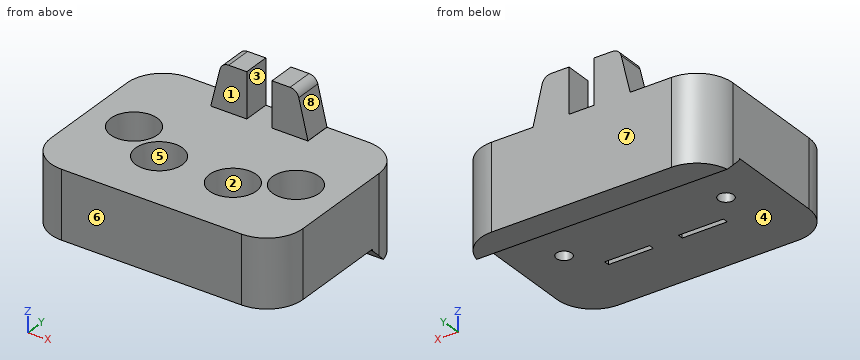
from build123d import *

# Parameters (mm, degrees)
SKETCH_W        = 35.56
SKETCH_H        = 25.4
SKETCH_R        = 1.0795
SKETCH_W_2      = 6.35
SKETCH_H_2      = 0.762
PAD_DEPTH       = 1.905
SKETCH001_W     = 35.56
SKETCH001_H     = 25.4
PAD001_DEPTH    = 7.62
SKETCH002_R     = 3.302
POCKET_DEPTH    = 7.62
SKETCH003_W     = 35.56
SKETCH003_H     = 6.35
PAD002_DEPTH    = 2.54
SKETCH004_W     = 5.08
SKETCH004_H     = 3.81
PAD003_DEPTH    = 6.35
CHAMFER_1_SIZE2 = 1.524
CHAMFER_1_SIZE  = 6.3246
CHAMFER_2_SIZE2 = 1.524
CHAMFER_2_SIZE  = 6.3246
FILLET_R        = 1.27
FILLET001_R     = 5.08
CHAMFER001_SIZE = 2.286


with BuildPart() as part:
    # Sketch → Pad (new body)
    with BuildSketch(Plane.XY):
        Rectangle(SKETCH_W, SKETCH_H)
        with Locations((-11.43, 0)):
            Circle(SKETCH_R, mode=Mode.SUBTRACT)
        with Locations((11.43, 0)):
            Circle(SKETCH_R, mode=Mode.SUBTRACT)
        with Locations((5.207, -4.191)):
            Rectangle(SKETCH_W_2, SKETCH_H_2, mode=Mode.SUBTRACT)
        with Locations((-5.207, -4.191)):
            Rectangle(SKETCH_W_2, SKETCH_H_2, mode=Mode.SUBTRACT)
    extrude(amount=PAD_DEPTH)

    # Sketch001 (on Face16 of Pad) → Pad001 (join)
    with BuildSketch(Plane.XY.offset(1.905)):
        Rectangle(SKETCH001_W, SKETCH001_H)
    extrude(amount=PAD001_DEPTH)

    # Sketch002 (on Face17 of Pad001) → Pocket (cut)
    with BuildSketch(Plane.XY.offset(9.525)):
        with Locations((-5.207, -3.81)):
            Circle(SKETCH002_R)
        with Locations((5.207, -3.81)):
            Circle(SKETCH002_R)
        with Locations((11.43, 0)):
            Circle(SKETCH002_R)
        with Locations((-11.43, 0)):
            Circle(SKETCH002_R)
    extrude(amount=-POCKET_DEPTH, mode=Mode.SUBTRACT)

    # Sketch003 (on Face1 of Pocket) → Pad002 (join)
    with BuildSketch(Plane(origin=(0, 0, 0), x_dir=(1, 0, 0), z_dir=(0, 0, -1))):
        with Locations((0, -9.525)):
            Rectangle(SKETCH003_W, SKETCH003_H)
    extrude(amount=PAD002_DEPTH)

    # Sketch004 (on Face15 of Pad002) → Pad003 (join)
    with BuildSketch(Plane.XY.offset(9.525)):
        with Locations((-4.318, 10.795)):
            Rectangle(SKETCH004_W, SKETCH004_H)
        with Locations((4.318, 10.795)):
            Rectangle(SKETCH004_W, SKETCH004_H)
    extrude(amount=PAD003_DEPTH)

    # Chamfer 1
    chamfer_1_edges = [part.edges().sort_by_distance(p)[0] for p in [
        (-6.858, 10.795, 15.875),
    ]]
    chamfer_1_side = part.faces().sort_by_distance((-6.858, 10.795, 12.7))[0]
    chamfer(chamfer_1_edges, length=CHAMFER_1_SIZE, length2=CHAMFER_1_SIZE2, reference=chamfer_1_side)

    # Chamfer 2
    chamfer_2_edges = [part.edges().sort_by_distance(p)[0] for p in [
        (6.858, 10.795, 15.875),
    ]]
    chamfer_2_side = part.faces().sort_by_distance((6.858, 10.795, 12.7))[0]
    chamfer(chamfer_2_edges, length=CHAMFER_2_SIZE, length2=CHAMFER_2_SIZE2, reference=chamfer_2_side)

    # Fillet
    fillet_edges = [part.edges().sort_by_distance(p)[0] for p in [
        (-5.334, 10.795, 15.875),
        (5.334, 10.795, 15.875),
    ]]
    fillet(fillet_edges, radius=FILLET_R)

    # Fillet001
    fillet001_edges = [part.edges().sort_by_distance(p)[0] for p in [
        (-17.78, -12.7, 4.7625),
        (-17.78, 12.7, 3.4925),
        (17.78, -12.7, 4.7625),
        (17.78, 12.7, 3.4925),
    ]]
    fillet(fillet001_edges, radius=FILLET001_R)

    # Chamfer001
    chamfer001_edges = [part.edges().sort_by_distance(p)[0] for p in [
        (0, 6.35, -2.54),
    ]]
    chamfer(chamfer001_edges, length=CHAMFER001_SIZE)


solid = part.part
Design review of the part built by this model. Coordinates are the model's own, in mm. Face numbers are marked on the shaded views. A direction names the side the tool comes from. Coordinates: 2 decimals unless noted, no trailing zeros. Loops run counter-clockwise (first coordinate to the right, second up) from the corner with the lowest first, then second, coordinate; pieces in that order, holes last.
Item 1: Draft analysis for pull direction Y (two halves, no side actions). For the marked faces 5, 6, 7 and 8, state which applies: pulls with the +Y half, pulls with the -Y half, needs draft (parallel to the pull), parting line crosses it, or undercut.
Completed:
face 5: undercut
face 6: pulls with the -Y half
face 7: pulls with the +Y half
face 8: needs draft
Item 2: Add section B-B (z = 0.5). Write out the cut boundary in (x, y).
Completed:
outline: (-17.78, -7.62) arc R5.08 ccw to (-12.7, -12.7) - (12.7, -12.7) arc R5.08 ccw to (17.78, -7.62) - (17.78, 7.62) arc R5.08 ccw to (12.7, 12.7) - (-12.7, 12.7) arc R5.08 ccw to (-17.78, 7.62) - close; hole circle Ø2.16 at (-11.43, 0); hole (-8.38, -4.57) - (-2.03, -4.57) - (-2.03, -3.81) - (-8.38, -3.81) - close; hole (2.03, -4.57) - (8.38, -4.57) - (8.38, -3.81) - (2.03, -3.81) - close; hole circle Ø2.16 at (11.43, 0)
Item 3: Add section C-C (y = 0). Write out the cut boundary in (x, z) (1 decimal).
Completed:
outline: (-17.8, 0) - (-12.5, 0) - (-12.5, 1.9) - (-14.7, 1.9) - (-14.7, 9.5) - (-17.8, 9.5) - close; (-10.4, 0) - (10.4, 0) - (10.4, 1.9) - (8.1, 1.9) - (8.1, 9.5) - (-8.1, 9.5) - (-8.1, 1.9) - (-10.4, 1.9) - close; (12.5, 0) - (17.8, 0) - (17.8, 9.5) - (14.7, 9.5) - (14.7, 1.9) - (12.5, 1.9) - close
Item 4: For the marked faces 1, 2, 3 and 4, list the 3-axis set-ups (+Z, -Z, +X, -X, +Y, -Y) from which the entire face can be reached by the end or side of a thin tool; tool diameter is ignored.
Completed:
face 1: +Z, +X, -X, -Y
face 2: +Z
face 3: +Z, +Y, -Y
face 4: -Z, +X, -X, -Y
Item 5: Add section D-D (z = 11.5). Write out the cut boundary in (x, y), and give its area (3 significant figures).
Completed:
outline: (-6.39, 8.89) - (-1.78, 8.89) - (-1.78, 12.7) - (-6.39, 12.7) - close; (1.78, 8.89) - (6.39, 8.89) - (6.39, 12.7) - (1.78, 12.7) - close
area: 35.1 mm2
Item 6: Clearance check with flat-ended pins moving along their axes: pin 1 (12 mm diameter, centred on x = 7, y = -9.5, fed in from -Z); pin 2 (4 mm diameter, centred on x = -11.43, y = 0, fed in from +Z) (3 decimals); pin 3 (5 mm diameter, centred on x = -9, y = 1, fed in from +Z) (3 decimals); pin 4 (8 mm diameter, centred on y = -9, z = 12.5, fed in from +X). State where each tip first meets the part, or that it passes through.
Completed:
pin 1: stops at z = 0
pin 2: stops at z = 1.905
pin 3: stops at z = 9.525
pin 4: stops at x = 17.78
Item 7: Wall thickness on L1, parallel to X at y = -0.25, z = 7; L2, parallel to Y at x = -11.43, z = 0.95; L3, parallel to Z at x = -14, y = 9.5 (3 decimals): over which ranges is each line inside the solid? List them lowest first.
Completed:
L1: x = -17.78 to -14.72, -8.14 to 8.14, 14.72 to 17.78
L2: y = -12.7 to -1.08, 1.08 to 12.7
L3: z = -2.54 to 9.525
